Build history of the part. All positions in model axes, mm. A direction names the side the tool comes from. Round coordinates to 2 decimals unless told otherwise and drop trailing zeros. Write each loop counter-clockwise with the first axis right and the second up, starting at its lowest first coordinate (ties: lowest second). Pieces come first, ordered by that corner, then holes. Notation, with made-up numbers: (-31.75, -33) - (-13.75, -33) arc R12 cw to (-13.75, -19) - close; hole circle Ø6 at (-35, 41.25). An arc over 180 degrees is marked (long way). One line per question, with ' | ' between items.
from build123d import *

# Parameters (mm, degrees)
SKETCH2_OUTSIDE_W  = 15.626
SKETCH2_OUTSIDE_H  = 15.626
CUT_EXTRUDE1_DEPTH = 2.54
SKETCH3_R          = 1.27
CUT_EXTRUDE2_DEPTH = 11.43
SKETCH4_R          = 0.635
CUT_EXTRUDE3_DEPTH = 11.43


with BuildPart() as part:
    # Sketch1 → Revolve2 (revolve)
    with BuildSketch(Plane(origin=(0, 0, 0), x_dir=(0, 0, -1), z_dir=(1, 0, 0))):
        Polygon((0, 0), (0, 13.716), (2.032, 13.716), (2.839757444, 12.908242556), (2.839757444, 11.938), (2.032, 11.938), (2.032, 9.398), (4.868925194, 9.398), (4.868925194, 6.858), (2.794, 6.858), (2.794, 1.613116652), align=None)
    revolve(axis=Axis((0, 0, 0), (0, 1, 0)))

    # Sketch2 outside → Cut-Extrude1 (cut)
    with BuildSketch(Plane(origin=(0, 9.398, 0), x_dir=(1, 0, 0), z_dir=(0, 1, 0))):
        Rectangle(SKETCH2_OUTSIDE_W, SKETCH2_OUTSIDE_H)
        Polygon((3.366014334, -1.452852654), (2.941214474, 2.188627596), (-0.424799861, 3.64148025), (-3.366014334, 1.452852654), (-2.941214474, -2.188627596), (0.424799861, -3.64148025), align=None, mode=Mode.SUBTRACT)
    extrude(amount=-CUT_EXTRUDE1_DEPTH, mode=Mode.SUBTRACT)

    # Sketch3 → Cut-Extrude2 (cut)
    with BuildSketch(Plane(origin=(0, 13.716, 0), x_dir=(1, 0, 0), z_dir=(0, 1, 0))):
        Circle(SKETCH3_R)
    extrude(amount=-CUT_EXTRUDE2_DEPTH, mode=Mode.SUBTRACT)

    # Sketch4 → Cut-Extrude3 (cut)
    with BuildSketch(Plane(origin=(0, 0, 0), x_dir=(0, 0, -1), z_dir=(1, 0, 0))):
        with Locations((0, 3.79195236)):
            Circle(SKETCH4_R)
    extrude(amount=-CUT_EXTRUDE3_DEPTH, mode=Mode.SUBTRACT)


solid = part.part
Q1. Drill centre lines: L1, parallel to Z at x = 0, y = 11.25; L2, parallel to Z at x = 0, y = 5.75; L3, parallel to Y at x = -2.5, z = -0.5. Where is each one in solid material? Low to high. Write a range as from..to.
Found:
L1: -2.03..-1.27, 1.27..2.03 | L2: -2.79..-1.27, 1.27..2.79 | L3: 1.47..3.4, 4.18..9.4, 11.94..13.2
Q2. Which spindle directions (+Z, -Z, +X, -X, +Y, -Y) get a long thin tool onto all of the face, cutting with end or side? Do faces 1 (the flat face through (1, 9.398, -2)), 2 (the flat face through (1, 6.858, 3)), 3 (the cylindrical face through (-2.816, 12.416, 0.37)), 4 (the cylindrical face through (-1.935, 3.82, 0.634)). Say none if no direction does.
Found:
face 1: none | face 2: -Y | face 3: +Y | face 4: -X
Q3. Drop flat-ended pins along their axis: pin 1 (1.7 mm diameter, centred on x = 0.5, z = -1, fed in from -Y); pin 2 (4 mm diameter, centred on y = 10.5, z = -0.5, fed in from +X); pin 3 (1.7 mm diameter, centred on y = 3.79, z = 0, fed in from -X). Give the stop position or say it passes through.
Found:
pin 1: y = 0.15 | pin 2: x = 3.33 | pin 3: x = -2.79
Q4. Saw through at B-B, the plane x = -2.25. State how many separate pieces and enclosed holes the cut face has, then the cut area to 3 significant figures.
Found:
separate pieces: 2 | enclosed holes: 1 | area: 33.6 mm^2
Q5. Saw through at A-A, the plane y = 8.75. List the corners of the cut face in (x, z), then the cut area to 3 significant figures.
Found:
outline: (-3.37, -1.45) - (-0.42, -3.64) - (2.94, -2.19) - (3.37, 1.45) - (0.42, 3.64) - (-2.94, 2.19) - close; hole circle Ø2.54 at (0, 0) | area: 29.9 mm^2
Q6. Saw through at C-C, the plane y = 6.5. List the corners of the cut face in (x, z), then the cut area to 3 significant figures.
Found:
outline: circle Ø5.59 at (0, 0); hole circle Ø2.54 at (0, 0) | area: 19.5 mm^2
Q7. Pull direction X, two halves, no side cores. Call faces 5 (the flat face through (3.157, 8.146, -0.342)), 6 (the flat face through (0, 2.286, 0)), 7 (the cylindrical face through (1.984, 10.65, 0.44)), 8 (the cylindrical face through (1.21, 8.08, -0.38)): +X half, -X half, draft (parallel to the pull), parting line (faces both ways), or undercut.
Found:
face 5: +X half | face 6: undercut | face 7: parting line | face 8: undercut
